```python
from build123d import *

# Parameters (mm, degrees)
SKETCH1_R           = 650
BOSS_EXTRUDE1_DEPTH = 20
SKETCH2_W           = 33.859391453
SKETCH2_H           = 72.958055336
SKETCH2_W_2         = 44.858886192
SKETCH2_H_2         = 83.856653026
BOSS_EXTRUDE2_DEPTH = 750
SKETCH3_R           = 45
BOSS_EXTRUDE3_DEPTH = 1186.61916287
FILLET1_R           = 10
SKETCH4_W           = 183.78137906
SKETCH4_H           = 72.271116226
BOSS_EXTRUDE4_DEPTH = 60
SKETCH5_W           = 137.162690518
SKETCH5_H           = 87.847771894
CUT_EXTRUDE1_DEPTH  = 139
SKETCH6_R           = 10.058928829
CUT_EXTRUDE2_DEPTH  = 200


with BuildPart() as part:
    # Sketch1 → Boss-Extrude1 (new body)
    with BuildSketch(Plane(origin=(0, 0, 0), x_dir=(1, 0, 0), z_dir=(0, 1, 0))):
        with Locations(Location((0, 0, 0), (0, 0, 270))):
            Circle(SKETCH1_R)
    extrude(amount=BOSS_EXTRUDE1_DEPTH)

    # Sketch2 → Boss-Extrude2 (add)
    with BuildSketch(Plane(origin=(0, 20, 0), x_dir=(1, 0, 0), z_dir=(0, 1, 0))):
        with Locations((616.00396434, -36.479027668)):
            Rectangle(SKETCH2_W, SKETCH2_H)
        with Locations((616.00396434, 36.479027668)):
            Rectangle(SKETCH2_W, SKETCH2_H)
        with Locations((-609.974337352, -41.928326513)):
            Rectangle(SKETCH2_W_2, SKETCH2_H_2)
        with Locations((-609.974337352, 41.928326513)):
            Rectangle(SKETCH2_W_2, SKETCH2_H_2)
    extrude(amount=BOSS_EXTRUDE2_DEPTH)

    # Sketch3 → Boss-Extrude3 (add)
    with BuildSketch(Plane(origin=(-587.544894256, 0, 0), x_dir=(0, 0, -1), z_dir=(1, 0, 0))):
        with Locations(Location((0, 670, 0), (0, 0, 180))):
            Circle(SKETCH3_R)
    extrude(amount=BOSS_EXTRUDE3_DEPTH)

    # Fillet1
    fillet1_edges = [part.edges().sort_by_distance(p)[0] for p in [
        (616.00396434, 20, -72.958055336),
        (-609.974337352, 20, 83.856653026),
        (-587.544894256, 20, 0),
        (-632.403780448, 20, 0),
        (-609.974337352, 20, -83.856653026),
        (616.00396434, 20, 72.958055336),
        (632.933660066, 20, 0),
        (599.074268613, 20, 0),
    ]]
    fillet(fillet1_edges, radius=FILLET1_R)

    # Sketch4 → Boss-Extrude4 (add)
    with BuildSketch(Plane(origin=(0, 20, 0), x_dir=(1, 0, 0), z_dir=(0, 1, 0))):
        with Locations((0, -579.075005183)):
            Rectangle(SKETCH4_W, SKETCH4_H)
    extrude(amount=BOSS_EXTRUDE4_DEPTH)

    # Sketch5 → Cut-Extrude1 (cut)
    with BuildSketch(Plane.XY.offset(615.210563296)):
        with Locations((0, 80)):
            Rectangle(SKETCH5_W, SKETCH5_H)
    extrude(amount=-CUT_EXTRUDE1_DEPTH, mode=Mode.SUBTRACT)

    # Sketch6 → Cut-Extrude2 (cut)
    with BuildSketch(Plane(origin=(91.89068953, 0, 0), x_dir=(0, 0, -1), z_dir=(1, 0, 0))):
        with Locations((-581.015384382, 64.297210262)):
            Circle(SKETCH6_R)
    extrude(amount=-CUT_EXTRUDE2_DEPTH, mode=Mode.SUBTRACT)


solid = part.part
```
The listing builds one solid part. Answer for the finished solid, in the listing's coordinates (mm). A direction names the side the tool comes from. Round coordinates to 2 decimals unless told otherwise and drop trailing zeros. Loops run counter-clockwise (first coordinate to the right, second up) from the corner with the lowest first, then second, coordinate; pieces in that order, holes last. Notation, with made-up numbers: (69.25, 38.25) - (103.25, 38.25) arc R24 ccw to (103.25, 51.25) - close; hole circle Ø8 at (-32.75, 60). An arc over 180 degrees is marked (long way). Return JSON: item names as keys, results as strings. Group by question number.
1. Each of these flat-tipped pins is pushed along its axis until it touches: P1, Ø21.5, axis at x = -10.5, z = 593, coming from the +Y side; P2, Ø11.5, axis at x = -75.5, z = 567.5, coming from the +Y side; P3, Ø13, axis at y = 62.5, z = 566.5, coming from the +X side. Where does it stop, or does it pass through?
2. The mould has two halves that part along Y. Classify faces 6 (the flat face through (-1, 30, 615.211)), 7 (the flat face through (-587.545, 395, 1)), 8 (the flat face through (-610, 770, -1)): pulls with the +Y half, pulls with the -Y half, needs draft (parallel to the pull), parting line crosses it, or undercut.
3. The part is cut by section B-B on y = 425. Determine the outline of the cut face in (x, z).
4. The part is cut by section D-D on y = 670. Determine the outline of the cut face in (x, z).
5. Consider probe 1 along X at (y, z) = (57, 26); probe 2 along Y at (x, z) = (208, -4.5); probe 3 along Y at (x, z) = (-260.5, -543). Determine where each line is inside the solid, lowest interval first.
6. Which of the six approach directions +Z, -Z, +X, -X, +Y, -Y give full straight-line access (tool end or side, diameter ignored) to faces 1 (the flat face through (616, 395, 72.958)), 2 (the flat face through (68.581, 53, 580)), 3 (the flat face through (-632.404, 395, -1)), 4 (the flat face through (91.891, 50, 580)), 5 (the flat face through (616, 395, -72.958))?
7. The part is cut by section C-C on z = 0. Determine the outline of the cut face in (x, y), then the cut area to 3 significant figures.
8. The part is cut by section A-A on x = 0. Determine the outline of the cut face in (y, z), then the cut area to 3 significant figures.
Resolved:
{
 "1": {"P1": "stops at y = 36.08", "P2": "stops at y = 80", "P3": "stops at x = 91.89"},
 "2": {"face 6": "needs draft", "face 7": "undercut", "face 8": "pulls with the +Y half"},
 "3": {"outline": "(-632.4, -83.86) - (-587.54, -83.86) - (-587.54, 83.86) - (-632.4, 83.86) - close; (599.07, -72.96) - (632.93, -72.96) - (632.93, 72.96) - (599.07, 72.96) - close"},
 "4": {"outline": "(-632.4, -83.86) - (-587.54, -83.86) - (-587.54, -45) - (599.07, -45) - (599.07, -72.96) - (632.93, -72.96) - (632.93, 72.96) - (599.07, 72.96) - (599.07, 45) - (-587.54, 45) - (-587.54, 83.86) - (-632.4, 83.86) - close"},
 "5": {"probe 1": "x = -632.4 to -587.54, 599.07 to 632.93", "probe 2": "y = 0 to 20, 625.23 to 714.77", "probe 3": "y = 0 to 20"},
 "6": {"face 1": "+Z, +X, +Y", "face 2": "+Z, -Z, +Y", "face 3": "+Z, -Z, -X, +Y", "face 4": "+Z, -Z, +X, +Y", "face 5": "-Z, +X, +Y"},
 "7": {"outline": "(-650, 0) - (650, 0) - (650, 20) - (642.93, 20) arc R10 cw to (632.93, 30) - (632.93, 770) - (599.07, 770) - (599.07, 715) - (-587.54, 715) - (-587.54, 770) - (-632.4, 770) - (-632.4, 30) arc R10 cw to (-642.4, 20) - (-650, 20) - close; hole (-587.54, 30) arc R10 ccw to (-577.54, 20) - (589.07, 20) arc R10 ccw to (599.07, 30) - (599.07, 625) - (-587.54, 625) - close", "area": "192,000 mm²"},
 "8": {"outline": "(0, -650) - (20, -650) - (20, 542.94) - (36.08, 542.94) - (36.08, 615.21) - (20, 615.21) - (20, 650) - (0, 650) - close; circle Ø90 at (670, 0)", "area": "33,500 mm²"}
}
